Check sheet for the modelled part. Datum: model origin and axes. Units: mm. A direction names the side the tool comes from. Give positions to 0.01 mm unless a question says otherwise; leave off trailing zeros. Write each loop counter-clockwise with the first axis right and the second up, starting at its lowest first coordinate (ties: lowest second). Pieces come first, ordered by that corner, then holes. Notation, with made-up numbers: (-21.5, 48) - (13.5, 48) arc R21 cw to (13.5, 63) - close; hole circle Ø1 at (-17.5, -1.5). An arc over 180 degrees is marked (long way). Return JSON: item names as keys, results as strings. Group by question number.
```python
from build123d import *

# Parameters (mm, degrees)
SKETCH1_W           = 10
SKETCH1_H           = 10
BOSS_EXTRUDE1_DEPTH = 10
CUT_EXTRUDE1_DEPTH  = 1
CUT_EXTRUDE2_DEPTH  = 1
CUT_EXTRUDE3_DEPTH  = 1
SKETCH5_W           = 2.238729714
SKETCH5_H           = 2.608108567
CUT_EXTRUDE4_DEPTH  = 1
CUT_EXTRUDE5_DEPTH  = 1
CUT_EXTRUDE6_DEPTH  = 1


with BuildPart() as part:
    # Sketch1 → Boss-Extrude1 (new body)
    with BuildSketch(Plane(origin=(0, 0, 0), x_dir=(1, 0, 0), z_dir=(0, 1, 0))):
        with Locations((5, 5)):
            Rectangle(SKETCH1_W, SKETCH1_H)
    extrude(amount=BOSS_EXTRUDE1_DEPTH)

    # Sketch2 → Cut-Extrude1 (cut)
    with BuildSketch(Plane(origin=(0, 10, 0), x_dir=(1, 0, 0), z_dir=(0, 1, 0))):
        Polygon((1.465466964, 1.710070359), (1.465466964, 8.284227428), (2.964562162, 8.284227428), (4.557350811, 4.997148894), (6.462450959, 8.284227428), (7.608638796, 8.284227428), (7.608638796, 1.710070359), (6.608638796, 1.710070359), (6.608638796, 5.332883756), (5.000234573, 3.131087683), (3.532370524, 3.131087683), (2.465466964, 5.332883756), (2.465466964, 1.710070359), align=None)
    extrude(amount=-CUT_EXTRUDE1_DEPTH, mode=Mode.SUBTRACT)

    # Sketch3 → Cut-Extrude2 (cut)
    with BuildSketch(Plane(origin=(10, 0, 0), x_dir=(0, 0, -1), z_dir=(1, 0, 0))):
        Polygon((8.63868002, 8.189348455), (8.63868002, 1.575196843), (7.522328424, 1.575196843), (7.522328424, 3.574876892), (1.797107491, 3.574876892), (1.797107491, 8.189348455), (4.047324941, 8.189348455), (4.047324941, 7.203608146), (2.569618508, 7.203608146), (2.569618508, 4.882272649), (7.522328424, 4.882272649), (7.522328424, 8.189348455), align=None)
    extrude(amount=-CUT_EXTRUDE2_DEPTH, mode=Mode.SUBTRACT)

    # Sketch4 → Cut-Extrude3 (cut)
    with BuildSketch(Plane.XZ):
        Polygon((7.109235008, -8.151746998), (2.677244084, -8.151746998), (2.677244084, -7.107897794), (4.283200213, -7.107897794), (4.283200213, -3.06528113), (2.436930969, -3.06528113), (2.436930969, -1.906165647), (8.875026218, -1.906165647), (8.875026218, -3.55360609), (6.449771082, -3.55360609), (6.449771082, -7.107897794), (7.109235008, -7.107897794), align=None)
    extrude(amount=-CUT_EXTRUDE3_DEPTH, mode=Mode.SUBTRACT)

    # Sketch5 → Cut-Extrude4 (cut)
    with BuildSketch(Plane.ZY):
        Polygon((-1.636879665, 2.166406858), (-8.437777795, 2.166406858), (-8.437777795, 7.84825918), (-1.636879665, 7.84825918), (-1.636879665, 6.537193973), (-4.003754487, 6.537193973), (-4.003754487, 3.929085406), (-1.636879665, 3.929085406), align=None)
        with Locations((-6.156693587, 5.23313969)):
            Rectangle(SKETCH5_W, SKETCH5_H, mode=Mode.SUBTRACT)
    extrude(amount=-CUT_EXTRUDE4_DEPTH, mode=Mode.SUBTRACT)

    # Sketch6 → Cut-Extrude5 (cut)
    with BuildSketch(Plane(origin=(0, 0, -10), x_dir=(-1, 0, 0), z_dir=(0, 0, -1))):
        Polygon((-9, 9), (-1, 9), (-1, 8), (-4.5, 8), (-4.5, 1), (-5.5, 1), (-5.5, 8), (-9, 8), align=None)
    extrude(amount=-CUT_EXTRUDE5_DEPTH, mode=Mode.SUBTRACT)

    # Sketch7 → Cut-Extrude6 (cut)
    with BuildSketch(Plane.XY):
        with BuildLine():
            ThreePointArc((7, 5), (9, 3), (7, 1))
            Line((7, 1), (1, 1))
            Line((1, 1), (1, 9))
            Line((1, 9), (7, 9))
            ThreePointArc((7, 9), (9, 7), (7, 5))
        make_face()
        with BuildLine():
            Line((2, 8), (7, 8))
            ThreePointArc((7, 8), (8, 7), (7, 6))
            Line((7, 6), (2, 6))
            Line((2, 6), (2, 8))
        make_face(mode=Mode.SUBTRACT)
        with BuildLine():
            Line((7, 4), (2, 4))
            Line((2, 4), (2, 2))
            Line((2, 2), (7, 2))
            ThreePointArc((7, 2), (8, 3), (7, 4))
        make_face(mode=Mode.SUBTRACT)
    extrude(amount=-CUT_EXTRUDE6_DEPTH, mode=Mode.SUBTRACT)


solid = part.part
```
Item 1: Section check D-D on x = 1.25. Record the cut outline in (y, z).
Item 2: Section check C-C on z = -7.75. Record the cut outline in (x, y).
Item 3: Material ranges on line 1 along Y through (x, z) = (4.25, -0.25); line 2 along Y through (x, z) = (0.5, -6.75); line 3 along Z through (x, y) = (7.5, 9.25), recorded low to high. Write a range as from..to.
Item 4: Access from +Z, -Z, +X, -X, +Y, -Y to the whole of each face (thin tool, end or side, straight path). Record for faces 4 (the face through (4.9, 0.5, -8.152)), 5 (the face through (7.1, 9.5, -1.71)), 6 (the face through (0.5, 5.2, -5.037)), 7 (the face through (9.5, 4.9, -8.639)), 8 (the face through (1, 8.5, -9.5)).
Item 5: Section check A-A on x = 2.25. Record the cut outline in (y, z), plus the area to 3 significant figures.
Item 6: Section check B-B on y = 7. Record the cut outline in (x, z), plus the area to 3 significant figures.
Item 7: Mould release check, pull along Z, two halves, no side actions. Record for faces 1 (the face through (9.5, 6.5, -7.522)), 2 (the face through (8, 5, 0)), 3 (the face through (4.9, 10, -6.2)): +Z half, -Z half, draft (parallel to the pull), parting line (faces both ways), or undercut.
Reply:
{
 "1": {"outline": "(0, -10) - (8, -10) - (8, -9) - (9, -9) - (9, -10) - (10, -10) - (10, 0) - (9, 0) - (9, -1) - (1, -1) - (1, 0) - (0, 0) - close"},
 "2": {"outline": "(0, 0) - (2.68, 0) - (2.68, 1) - (7.11, 1) - (7.11, 0) - (10, 0) - (10, 1.58) - (9, 1.58) - (9, 8.19) - (10, 8.19) - (10, 10) - (7.61, 10) - (7.61, 9) - (6.15, 9) - (6.15, 10) - (3.22, 10) - (3.22, 9) - (1.47, 9) - (1.47, 10) - (0, 10) - (0, 7.85) - (1, 7.85) - (1, 2.17) - (0, 2.17) - close"},
 "3": {"line 1": "0..1, 2..4, 6..8, 9..10", "line 2": "0..2.17, 3.93..6.54, 7.85..10", "line 3": "-10..-8.28, -1.71..0"},
 "4": {"face 4": "-Y", "face 5": "+Y", "face 6": "-X", "face 7": "+X", "face 8": "-Z"},
 "5": {"outline": "(0, -10) - (8, -10) - (8, -9) - (9, -9) - (9, -10) - (10, -10) - (10, -8.28) - (9, -8.28) - (9, -1.71) - (10, -1.71) - (10, 0) - (9, 0) - (9, -1) - (8, -1) - (8, 0) - (6, 0) - (6, -1) - (4, -1) - (4, 0) - (2, 0) - (2, -1) - (1, -1) - (1, 0) - (0, 0) - close", "area": "88.4 mm²"},
 "6": {"outline": "(0, -10) - (4.5, -10) - (4.5, -9) - (5.5, -9) - (5.5, -10) - (10, -10) - (10, -8.64) - (9, -8.64) - (9, -7.52) - (10, -7.52) - (10, -2.57) - (9, -2.57) - (9, -1.8) - (10, -1.8) - (10, 0) - (9, 0) - (9, -1) - (8, -1) - (8, 0) - (2, 0) - (2, -1) - (1, -1) - (1, 0) - (0, 0) - (0, -1.64) - (1, -1.64) - (1, -8.44) - (0, -8.44) - close", "area": "88.3 mm²"},
 "7": {"face 1": "undercut", "face 2": "+Z half", "face 3": "draft"}
}
